Answer from the drawing. Dimensions are ordinates in mm from the lowest x, y and z of the part. Coordinates: 2 decimals unless noted, no trailing zeros. Loops run counter-clockwise (first coordinate to the right, second up) from the corner with the lowest first, then second, coordinate; pieces in that order, holes last. Notation, with made-up numbers: (-2, 10.5) -> (19, 10.5) arc R26 ccw to (19, 48.5) -> close; hole circle Ø2 at (-14.5, 68). An arc over 180 degrees is marked (long way). Answer as CSV lines item,"result".
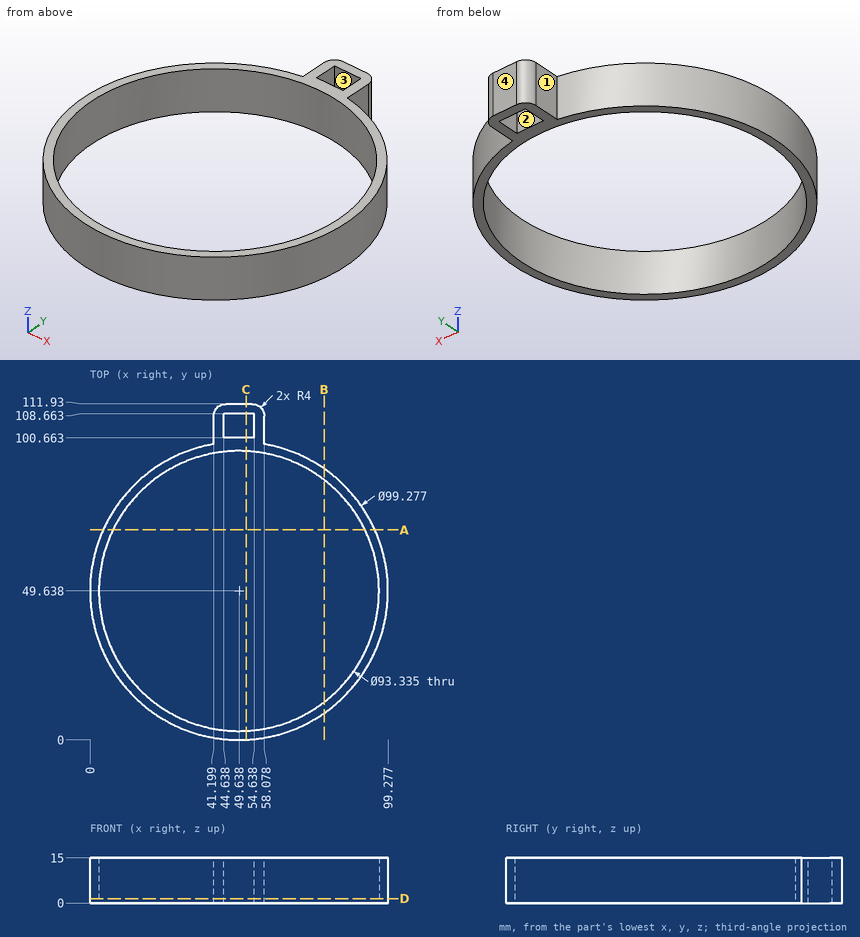
(1) For a pull along Y with two mould halves and no side action, classify the marked faces 1, 2, 3 and 4 as pulls with the +Y half, pulls with the -Y half, needs draft (parallel to the pull), parting line crosses it, or undercut.
Computed values:
face 1,"needs draft"
face 2,"undercut"
face 3,"undercut"
face 4,"pulls with the +Y half"
(2) A cutting plane is placed at A-A, the plane y = 70. Write down the section's boundary in (x, z).
Computed values:
outline,"(4.37, 0) -> (7.65, 0) -> (7.65, 15) -> (4.37, 15) -> close; (91.63, 0) -> (94.91, 0) -> (94.91, 15) -> (91.63, 15) -> close"
(3) A cutting plane is placed at C-C, the plane x = 52. Write down the section's boundary in (y, z).
Computed values:
outline,"(0.06, 0) -> (3.03, 0) -> (3.03, 15) -> (0.06, 15) -> close; (96.25, 0) -> (100.66, 0) -> (100.66, 15) -> (96.25, 15) -> close; (108.66, 0) -> (111.93, 0) -> (111.93, 15) -> (108.66, 15) -> close"
(4) A cutting plane is placed at D-D, the plane z = 1.5. Write down the section's boundary in (x, y) (1 decimal), and give its area (3 significant figures).
Computed values:
outline,"(41.2, 98.6) arc R49.6 ccw (long way) to (58.1, 98.6) -> (58.1, 107.9) arc R4 ccw to (54.1, 111.9) -> (45.2, 111.9) arc R4 ccw to (41.2, 107.9) -> close; hole circle Ø93.3 at (49.6, 49.6); hole (44.6, 100.7) -> (54.6, 100.7) -> (54.6, 108.7) -> (44.6, 108.7) -> close"
area,"1,030 mm2"
(5) Consider line 1 along Y through (x, z) = (49, 10.5) (1 decimal); line 2 along X through (y, z) = (105.5, 9.5); line 3 along X through (y, z) = (51, 2.75). Determine where each line is inside the solid, lowest interval first.
Computed values:
line 1,"0 to 3, 96.3 to 100.7, 108.7 to 111.9"
line 2,"41.2 to 44.64, 54.64 to 58.08"
line 3,"0.02 to 2.99, 96.29 to 99.26"
(6) A cutting plane is placed at B-B, the plane x = 78. Write down the section's boundary in (y, z).
Computed values:
outline,"(8.9, 0) -> (12.58, 0) -> (12.58, 15) -> (8.9, 15) -> close; (86.7, 0) -> (90.38, 0) -> (90.38, 15) -> (86.7, 15) -> close"
(7) Flat-ended cylindrical pins translate along their axes: pin 1 Ø2 at (x, z) = (43, 8) entering from -Y; pin 2 Ø6.5 at (y, z) = (104.5, 6.5) entering from -X; pin 3 Ø6 at (x, z) = (85.5, 9) entering from +Y. Find the tip coordinate at first contact, or state that the pin passes through.
Computed values:
pin 1,"y = 0.32"
pin 2,"x = 41.2"
pin 3,"y = 86.84"
